Autodesk Inventor part; units mm, degrees
ref_plane "WorkPlane1" through (0, 0, 0) normal (0, 0, 1) x (1, 0, 0)
ref_plane "MSC_PF1" through (0, 0, 0) normal (1, 0, 0) x (0, 1, 0)
ref_plane "MSC_PT1" through (0, 0, 0) normal (0, 0, -1) x (-1, 0, 0)
ref_plane "WorkPlane1" through (0, 0, 0) normal (0, 0, 1) x (1, 0, 0)
sketch "Sketch1" plane through (0, 0, 0) normal (0, 0, 1) x (1, 0, 0)
  point P0 (0, 0)
sketch "Sketch2" plane through (0, 0, 0) normal (0, 0, 1) x (1, 0, 0)
  line L0 (-8, 4.6189) -> (-8, -4.6189)
  line L1 (0, 9.2375) -> (-8, 4.6189)
  line L2 (8, 4.6189) -> (0, 9.2375)
  line L3 (8, -4.6189) -> (8, 4.6189)
  line L4 (0, -9.2375) -> (8, -4.6189)
  line L5 (-8, -4.6189) -> (0, -9.2375)
  circle A0 centre (0, 0) radius 8 construction
  dimension "d1" = 16
  dimension "d29" = 0
  dimension "d30" = 0
extrude "Extrusion1" add sketch "Sketch2" along normal blind 6.4
sketch "Sketch3" plane through (0, 0, 0) normal (1, 0, 0) x (0, 1, 0)
  line L0 (8, 6.4) -> (9.3375, 6.4)
  line L1 (9.3375, 5.6278) -> (8, 6.4)
  line L2 (9.3375, 6.4) -> (9.3375, 5.6278)
  line L3 (0, -1.28) -> (0, 7.68)
  line L4 (9.2375, 0) -> (9.2375, 6.4)
  dimension "d25" = 0.1
  dimension "d26" = 0
  dimension "d27" = 60
  dimension "d28" = 8
revolve "Revolution1" cut sketch "Sketch3" angle 360 about axis through (0, 0, -10) along (0, 0, 1)
sketch "Sketch4" plane through (0, 0, 0) normal (1, 0, 0) x (0, 1, 0)
  line L0 (0, -70) -> (0, 0)
  line L1 (-5, -70) -> (0, -70)
  line L2 (-5, 0) -> (-5, -70)
  line L3 (0, 0) -> (-5, 0)
  line L4 (0, -70) -> (0, 0)
  line L5 (-6, 0) -> (1, 0)
  line L6 (0, -84) -> (0, 14)
  dimension "d18" = 5
  dimension "d20" = 70
  dimension "d33" = 0
  dimension "d34" = 0
revolve "Revolution2" add sketch "Sketch4" angle 360 about axis through (0, 0, -70) along (0, 0, -1)
chamfer "Chamfer1" distance 0.75 angle 45 1 edges at (0, 5, -70)
fillet "Fillet1" radius 0.4 1 edges at (0, 5, 0)
thread "Thread1"
ref_plane "MSC_PF1" through (0, 0, 0) normal (1, 0, 0) x (0, 1, 0)
ref_plane "MSC_PT1" through (0, 0, 0) normal (0, 0, -1) x (-1, 0, 0)
equation "\"d22\" = 0.5 * PTC"
equation "\"d23\" = 0.5 * PTC"
equation "\"d24\" = r"
equation "\"d1\" = ParS"
equation "\"d6\" = ParK"
equation "\"b\" = NLG - 2 * PTC"
equation "\"d28\" = 0.5 * ParS"
equation "\"d18\" = 0.5 * NND"
equation "\"d20\" = NLG"
equation "\"NLG\" = 70"
equation "\"PTC\" = 1.5"
equation "\"ParK\" = 6.4"
equation "\"ParS\" = 16"
equation "\"msp_es\" = 0.577367 * ParS"
equation "\"r\" = 0.4"
equation "\"K1\" = 4.17"
properties part number "DIN EN ISO 4018 - M10x70" material "Stainless Steel"
Here's how the part is built. I have some questions about the finished solid (model axes, mm). A direction names the side the tool comes from. Coordinates: 2 decimals unless noted, no trailing zeros. Order: outer loops, then holes, each group sorted by start corner. A loop starts at its lowest first (then second) coordinate and runs counter-clockwise, first axis right, second up.
1) Will these pins go through, and if not, where does the flat tip stop? pin 1 (5 mm diameter, centred on x = -1, z = -5, fed in from +Y); pin 2 (2 mm diameter, centred on y = -1.5, z = -46, fed in from -X); pin 3 (1.5 mm diameter, centred on y = 5, z = -45.5, fed in from -X); pin 4 (1.5 mm diameter, centred on y = -6.5, z = -38, fed in from -X).
2) Imagine slicing it at B-B on z = -36.5. List the corners of the cut face in (x, y) for me, and give its area (3 significant figures).
3) Imagine slicing it at A-A on z = 2. List the corners of the cut face in (x, y) for me.
4) I need wall thicknesses on line 1 (Z direction, x = 4.5, y = -3.75); line 2 (X direction, y = -0.25, z = -64); line 3 (X direction, y = 2, z = -58.5). Which ranges of each line are inside material? Lowest first, please.
5) Which directions (+Z, -Z, +X, -X, +Y, -Y) give clear straight access to the entire face, cutting with the end or side of a thin tool? Please do faces 1 (the face through (7.179, 4.168, 6.226)), 2 (the face through (4.88, 1.08, -35.31)).
Response values:
1. pin 1: stops at y = 5
1. pin 2: stops at x = -4.97
1. pin 3: stops at x = -2.63
1. pin 4: passes through
2. outline: circle Ø10 at (0, 0)
2. area: 78.5 mm2
3. outline: (-8, -4.62) - (0, -9.24) - (8, -4.62) - (8, 4.62) - (0, 9.24) - (-8, 4.62) - close
4. line 1: z = 0 to 6.4
4. line 2: x = -4.99 to 4.99
4. line 3: x = -4.58 to 4.58
5. face 1: +Z, +X, +Y
5. face 2: -Z
